Part model, mm, in its own coordinate system. Face numbers are marked on the shaded views. A direction names the side the tool comes from. Coordinates: 2 decimals unless noted, no trailing zeros. Order: outer loops, then holes, each group sorted by start corner. A loop starts at its lowest first (then second) coordinate and runs counter-clockwise, first axis right, second up.
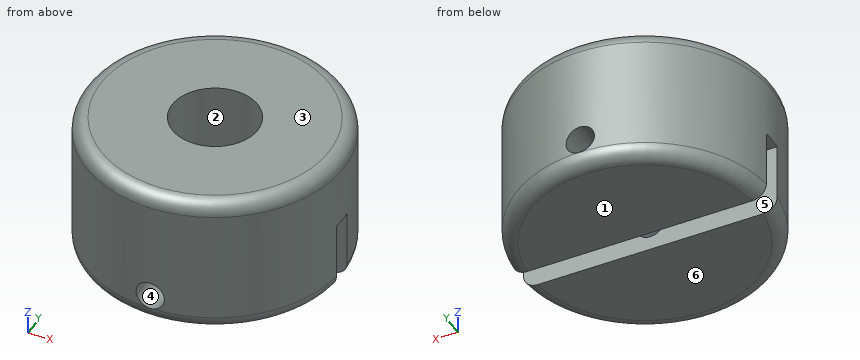
```python
from build123d import *

# Parameters (mm, degrees)
SKETCH_1_R               = 9
EXTRUDE_1_DEPTH          = 10
CUT_EXTRUDE_1_DEPTH      = 17.186414056
CUT_EXTRUDE_1_DEPTH_BACK = 17.186414056
SKETCH_2_W               = 10
SKETCH_2_H               = 1.5
CUT_EXTRUDE_2_DEPTH      = 17.186414056
CUT_EXTRUDE_2_DEPTH_BACK = 17.186414056
SKETCH_3_R               = 1
FILLET_1_R               = 1
SKETCH_4_R               = 3
CUT_EXTRUDE_3_DEPTH      = 6


with BuildPart() as part:
    # 草图1 → 凸台-拉伸1 (new body)
    with BuildSketch(Plane.XY):
        Circle(SKETCH_1_R)
    extrude(amount=EXTRUDE_1_DEPTH)

    # 草图2 → 切除-拉伸1 (cut, two sides: drawn at the far end of the back side and taken through both)
    with BuildSketch(Plane(origin=(0, 0, 0), x_dir=(0, 0, -1), z_dir=(1, 0, 0)).offset(-CUT_EXTRUDE_1_DEPTH_BACK)):
        Rectangle(SKETCH_2_W, SKETCH_2_H)
    extrude(amount=CUT_EXTRUDE_1_DEPTH + CUT_EXTRUDE_1_DEPTH_BACK, mode=Mode.SUBTRACT)

    # 草图3 → 切除-拉伸2 (cut, two sides: drawn at the far end of the back side and taken through both)
    with BuildSketch(Plane(origin=(0, 0, 0), x_dir=(1, 0, 0), z_dir=(0, 1, 0)).offset(-CUT_EXTRUDE_2_DEPTH_BACK)):
        with Locations(Location((0, -2, 0), (0, 0, 270))):
            Circle(SKETCH_3_R)
    extrude(amount=CUT_EXTRUDE_2_DEPTH + CUT_EXTRUDE_2_DEPTH_BACK, mode=Mode.SUBTRACT)

    # 圆角1
    fillet_1_edges = [part.edges().sort_by_distance(p)[0] for p in [
        (-9, 0, 10),
        (0, 9, 0),
        (0, -9, 0),
    ]]
    fillet(fillet_1_edges, radius=FILLET_1_R)

    # 草图4 → 切除-拉伸3 (cut)
    with BuildSketch(Plane.XY.offset(10)):
        Circle(SKETCH_4_R)
    extrude(amount=-CUT_EXTRUDE_3_DEPTH, mode=Mode.SUBTRACT)


solid = part.part
```
(1) Tool access for the marked faces 1 and 2: list every direction of +Z, -Z, +X, -X, +Y, -Y with a clear straight run to the whole face (end or side of a thin tool).
(2) Drop flat-ended pins along their axis: pin 1 (5 mm diameter, centred on y = -3, z = 5, fed in from -X); pin 2 (4 mm diameter, centred on x = -4, z = 3, fed in from -Y); pin 3 (6 mm diameter, centred on y = -4.5, z = 3, fed in from +X). Give the stop position or say it passes through.
(3) Slice it at C-C, the plane z = 8.5. Give the cut face in (x, y).
(4) Probe line 1 (Y direction, x = 0.75, z = 2.75); line 2 (Y direction, x = 0, z = 8.2); line 3 (Z direction, x = 0, y = -7). List the from-to ranges inside material, lowest first.
(5) Pull direction Z, two halves, no side cores. Call the marked faces 3, 4, 5 and 6: +Z half, -Z half, draft (parallel to the pull), parting line (faces both ways), or undercut.
(6) Slice it at B-B, the plane z = 2. Give the cut face in (x, y).
(7) Slice it at A-A, the plane y = 0. Give the cut face in (x, z).
Here are the results:
1. face 1: -Z, +X, -X, +Y, -Y
1. face 2: +Z
2. pin 1: stops at x = -8.99
2. pin 2: stops at y = -8.77
2. pin 3: stops at x = 8.87
3. outline: circle Ø18 at (0, 0); hole circle Ø6 at (0, 0)
4. line 1: y = -8.97 to -0.75, 0.75 to 8.97
4. line 2: y = -9 to -3, 3 to 9
4. line 3: z = 0 to 1, 3 to 10
5. face 3: +Z half
5. face 4: undercut
5. face 5: draft
5. face 6: -Z half
6. outline: (-8.97, -0.75) arc R9 ccw to (-1, -8.94) - (-1, -0.75) - close; (-8.97, 0.75) - (-1, 0.75) - (-1, 8.94) arc R9 ccw to start; (1, -8.94) arc R9 ccw to (8.97, -0.75) - (1, -0.75) - close; (1, 0.75) - (8.97, 0.75) arc R9 ccw to (1, 8.94) - close
7. outline: (-9, 5) - (-3, 5) - (-3, 10) - (-8, 10) arc R1 ccw to (-9, 9) - close; (3, 5) - (9, 5) - (9, 9) arc R1 ccw to (8, 10) - (3, 10) - close
